Autodesk Inventor part; units mm, degrees
ref_plane "Work Plane1" through (29, 0, 0) normal (0, -1, 0) x (1, 0, 0)
ref_plane "YZ Plane" through (0, 0, 0) normal (1, 0, 0) x (0, 1, 0)
ref_plane "XZ Plane" through (0, 0, 0) normal (0, 1, 0) x (-1, 0, 0)
sketch "Skizze1" plane through (0, 0, 0) normal (0, 0, 1) x (1, 0, 0)
  line L0 (0.2, 0) -> (8, 0)
  line L1 (8, 0) -> (8, 2.5)
  line L2 (8, 2.5) -> (2.4, 2.5)
  line L3 (2.4, 2.5) -> (1.9091, 2.5)
  line L4 (1.9091, 2.5) -> (0, 2.5)
  line L5 (0, 2.5) -> (0, 4.25)
  line L6 (0, 4.25) -> (-3.5, 4.25)
  line L7 (-3.5, 4.25) -> (-3.5, 1.7321)
  line L8 (-3.5, 1.7321) -> (-0.8, 1.7321)
  line L9 (-0.8, 1.7321) -> (0.2, 0)
  line L10 (-5.8, 0) -> (10.3, 0)
  line L11 (0, -0.85) -> (0, 5.1)
  line L12 (2.4, 2.5) -> (0, 2.5) construction
  dimension "d1" = 5.6
  dimension "d2" = 0.4909
  dimension "d3" = 3.5
  dimension "d4" = 2.7
  dimension "d5" = 60
  dimension "d6" = 5
  dimension "d7" = 5
  dimension "d8" = 3.4641
  dimension "d9" = 8.5
  dimension "d26" = 8
revolve "Körper" add sketch "Skizze1" angle 360 about axis through (0.2, 0, 0) along (1, 0, 0) contours L9 L11 L4 L3 L2 L1 L0 | L9 L8 L7 L6 L5 L11
sketch "Skizze2" plane through (-3.5, 0, 0) normal (-1, 0, 0) x (0, 0, 1)
  circle A0 centre (0, 0) radius 1.7321
  line L0 (0, -5.95) -> (0, 5.95)
  line L1 (-5.95, 0) -> (5.95, 0)
  line L2 (1.7321, 0) -> (0.866, -1.5)
  line L3 (0.866, -1.5) -> (-0.866, -1.5)
  line L4 (-0.866, -1.5) -> (-1.7321, 0)
  line L5 (-1.7321, 0) -> (-0.866, 1.5)
  line L6 (-0.866, 1.5) -> (0.866, 1.5)
  line L7 (0.866, 1.5) -> (1.7321, 0)
extrude "Loch" add sketch "Skizze2" against normal up to next contours L7 A0 | A0 L2 | L6 L0 A0 | A0 L0 L3 | L0 L6 A0 | A0 L3 L0 | L4 A0 | A0 L5
fillet "Rundung1" radius 0.5 1 edges at (-3.5, -4.25, 0)
thread "Gewinde"
chamfer "Fase1" distance 0.4908 distance2 0.4908 1 edges at (8, -2.5, 0) measured on face at (8, -0.6238, -0.819)
ref_plane "Work Plane1" through (29, 0, 0) normal (0, -1, 0) x (1, 0, 0)
fillet "Fillet2" radius 0.1 1 edges at (0, -2.5, 0)
equation "\"d1\" = GEL"
equation "\"d3\" = KOH"
equation "\"d4\" = INTI"
equation "\"d6\" = GD"
equation "\"d7\" = BDM"
equation "\"d8\" = 1.1547 * SW"
equation "\"d9\" = KOD"
equation "\"d26\" = NLG"
equation "\"d30\" = R"
equation "\"d17\" = RR"
equation "\"d13\" = GEL"
equation "\"d15\" = -0.5 * SPD + 0.5 * GD"
equation "\"d16\" = GUL"
equation "\"GD\" = NND"
equation "\"NLG\" = 8"
equation "\"GEL\" = 5.6"
equation "\"KOD\" = 8.5"
equation "\"KOH\" = 3.5"
equation "\"INTI\" = 2.7"
equation "\"GAL\" = 0.61345 * PTC"
equation "\"GUL\" = 0.61345 * PTC"
equation "\"BDM\" = NND"
equation "\"SW\" = 3"
equation "\"RR\" = 0.5"
equation "\"SPD\" = NND - 1.2269 * PTC"
equation "\"R\" = 0.1"
equation "\"TOA\" = 30deg"
equation "\"GD1\" = THREADDIA - 1.2269 * PTC"
equation "\"THREADDIA\" = 5"
equation "\"FAWI\" = 45deg"
equation "\"ANG\" = 120deg"
equation "\"PTC\" = 0.8"
equation "\"NND\" = 5"
equation "\"E0\" = 1.155 * SW"
properties part number "DIN 7984 - M5 x 8" material "Stahl, weich"
The model under review builds one solid part; all positions refer to its coordinate system, in mm. A direction names the side the tool comes from. Give positions to 0.01 mm unless a question says otherwise; leave off trailing zeros. Loops run counter-clockwise (first coordinate to the right, second up) from the corner with the lowest first, then second, coordinate; pieces in that order, holes last. Notation, with made-up numbers: (55.25, -11) - (86.25, -11) arc R20 cw to (86.25, 22) - close; hole circle Ø6 at (-39.75, -15.5). An arc over 180 degrees is marked (long way). Answer as a JSON object with one key per item and string values.
Q1. Add section B-B on x = 2.5. State the section outline as (y, z) points, plus the area to 3 significant figures.
Worked out:
{"outline": "circle Ø5 at (0, 0)", "area": "19.6 mm^2"}
Q2. To check wall thickness, follow line 1 along X through (y, z) = (-0.5, 3.75); line 2 along Y through (x, z) = (3, -2). State the ranges of each line that lie inside material, in increasing order.
Worked out:
{"line 1": "x = -3.5 to 0", "line 2": "y = -1.5 to 1.5"}
Q3. Add section A-A on x = -2. State the section outline as (y, z) points.
Worked out:
{"outline": "circle Ø8.5 at (0, 0); hole (-1.5, -0.87) - (0, -1.73) - (1.5, -0.87) - (1.5, 0.87) - (0, 1.73) - (-1.5, 0.87) - close"}
Q4. Insertion check: pin 1 (1 mm diameter, centred on x = 1, y = 1, fed in from +Z); pin 2 (2 mm diameter, centred on x = 2, y = 1.5, fed in from -Z). Each pin has a flat end and moves straight along its axis. Give the tip position at first contact, or say it passes through.
Worked out:
{"pin 1": "stops at z = 2.45", "pin 2": "stops at z = -2.45"}
Q5. For faces 4 (the flat face through (-2, 1.5, 0)), 5 (the flat face through (8, 0, 0)), 6 (the flat face through (0, 2, 2)), list the 3-axis set-ups (+Z, -Z, +X, -X, +Y, -Y) from which the entire face can be reached by the end or side of a thin tool; tool diameter is ignored.
Worked out:
{"face 4": "-X", "face 5": "+Z, -Z, +X, +Y, -Y", "face 6": "+X"}
Q6. Mouldability with a two-part tool opening along Y and no side actions: class faces 1 (the flat face through (-3.5, -2, 0)), 2 (the cylindrical face through (-1.521, 2.285, -3.584)), 3 (the flat face through (-2.103, -0.74, 1.305)) as +Y half, -Y half, draft (parallel to the pull), parting line (faces both ways), or undercut.
Worked out:
{"face 1": "draft", "face 2": "parting line", "face 3": "undercut"}
Q7. Add section C-C on x = -0.25. State the section outline as (y, z) points.
Worked out:
{"outline": "circle Ø8.5 at (0, 0); hole circle Ø1.56 at (0, 0)"}
